Part model, mm, in its own coordinate system. Give positions to 0.01 mm unless a question says otherwise; leave off trailing zeros. Write each loop counter-clockwise with the first axis right and the second up, starting at its lowest first coordinate (ties: lowest second). Pieces come first, ordered by that corner, then holes. Notation, with made-up numbers: M -1,-4.75 L 41,-4.75 A23 cw 41,10.25 Z; hole C -3.75,-6.5 d11. An arc over 180 degrees is marked long. Use a Markdown table: item, result.
```python
from build123d import *

# Parameters (mm, degrees)
F0_R     = 4.222035
F1_DEPTH = 6
F2_DEPTH = 3
F3_SIZE  = 1.5
F4_R     = 1


with BuildPart() as f1:
    # F0 (on Top) → F1 (new body)
    with BuildSketch(Plane.XY):
        with BuildLine():
            Line((31.328976, 34.585057), (-13.897816, 34.585057))
            ThreePointArc((-13.897816, 34.585057), (-27.394685, 43.53433), (-18.671024, 29.890551))
            Line((-18.671024, 29.890551), (-18.671024, -15.414943))
            Line((-18.671024, -15.414943), (31.328976, -15.414943))
            Line((31.328976, -15.414943), (31.328976, 34.585057))
        make_face()
        Polygon((-10.122895, 2.46298), (-0.055609, -7.604307), (-9.207687, -8.519513), (-11.86179, -6.414536), align=None, mode=Mode.SUBTRACT)
        Polygon((11.018406, -7.146703), (-9.685952, 24.921147), (-4.439394, 26.535474), (22.275463, -2.113059), (19.833142, -8.3599), align=None, mode=Mode.SUBTRACT)
        with Locations((-21.591602, 37.633959)):
            Circle(F0_R, mode=Mode.SUBTRACT)
        Polygon((24.128397, 12.799296), (10.983175, 24.906736), (21.130362, 25.598589), (24.704942, 22.254631), align=None, mode=Mode.SUBTRACT)
    extrude(amount=F1_DEPTH)

    # F0 (on Top) → F2 (join)
    with BuildSketch(Plane.XY):
        with BuildLine():
            Line((31.328976, 34.585057), (-13.897816, 34.585057))
            ThreePointArc((-13.897816, 34.585057), (-27.394685, 43.53433), (-18.671024, 29.890551))
            Line((-18.671024, 29.890551), (-18.671024, -15.414943))
            Line((-18.671024, -15.414943), (31.328976, -15.414943))
            Line((31.328976, -15.414943), (31.328976, 34.585057))
        make_face()
        Polygon((-10.122895, 2.46298), (-0.055609, -7.604307), (-9.207687, -8.519513), (-11.86179, -6.414536), align=None, mode=Mode.SUBTRACT)
        Polygon((11.018406, -7.146703), (-9.685952, 24.921147), (-4.439394, 26.535474), (22.275463, -2.113059), (19.833142, -8.3599), align=None, mode=Mode.SUBTRACT)
        with Locations((-21.591602, 37.633959)):
            Circle(F0_R, mode=Mode.SUBTRACT)
        Polygon((24.128397, 12.799296), (10.983175, 24.906736), (21.130362, 25.598589), (24.704942, 22.254631), align=None, mode=Mode.SUBTRACT)
        Polygon((-4.439394, 26.535474), (-9.685952, 24.921147), (11.018406, -7.146703), (19.833142, -8.3599), (22.275463, -2.113059), align=None)
        Polygon((21.130362, 25.598589), (10.983175, 24.906736), (24.128397, 12.799296), (24.704942, 22.254631), align=None)
        Polygon((-9.207687, -8.519513), (-0.055609, -7.604307), (-10.122895, 2.46298), (-11.86179, -6.414536), align=None)
    extrude(amount=F2_DEPTH)

    # F3
    f3_edges = [f1.edges().sort_by_distance(p)[0] for p in [
        (8.918034, 12.211207, 6),
        (-7.062673, 25.72831, 6),
        (0.666227, 8.887222, 6),
        (15.425774, -7.753301, 6),
        (21.054302, -5.23648, 6),
        (22.917652, 23.92661, 6),
        (16.056768, 25.252663, 6),
        (17.555786, 18.853016, 6),
        (24.416669, 17.526963, 6),
        (-5.089252, -2.570663, 6),
        (-10.992342, -1.975778, 6),
        (-10.534738, -7.467025, 6),
        (-4.631648, -8.06191, 6),
    ]]
    chamfer(f3_edges, length=F3_SIZE)

    # F4
    f4_edges = [f1.edges().sort_by_distance(p)[0] for p in [
        (31.328976, 9.585057, 6),
        (6.328976, -15.414943, 6),
        (8.71558, 34.585057, 6),
        (-18.671024, 7.237804, 6),
        (-18.671024, -15.414943, 3),
        (31.328976, -15.414943, 3),
        (31.328976, 34.585057, 3),
    ]]
    fillet(f4_edges, radius=F4_R)


solid = f1.part
```
1. Drill centre lines: L1, parallel to X at y = -4.5, z = 3.75; L2, parallel to Y at x = -3, z = 1; L3, parallel to Z at x = -7.5, y = -5.5. Where is each one in solid material? Low to high.
Findings below:
| item | result |
|---|---|
| L1 | -18.67 to -11.49, -3.16 to 9.31, 21.34 to 31.33 |
| L2 | -15.41 to 34.59 |
| L3 | 0 to 3 |
2. Drop flat-ended pins along their axis: P1, Ø2, axis at y = 12.5, z = 3.5, coming from the -X side; P2, Ø3.5, axis at x = -8.5, y = -4.5, coming from the +Z side; P3, Ø3, axis at x = 6, z = 2.5, coming from the +Y side. Give the stop position or say it passes through.
Findings below:
| item | result |
|---|---|
| P1 | x = -18.67 |
| P2 | z = 3 |
| P3 | y = 34.59 |
3. Cut at B-B, the plane z = 3.75. Give the cut face in (x, y).
Findings below:
| item | result |
|---|---|
| outline | M -18.67,-14.41 A1 ccw -17.67,-15.41 L 30.33,-15.41 A1 ccw 31.33,-14.41 L 31.33,33.59 A1 ccw 30.33,34.59 L -13.9,34.59 A8.28 ccw long -18.67,29.89 Z; hole C -21.59,37.63 d8.44; hole M -11.86,-6.41 L -9.21,-8.52 L -0.06,-7.6 L -10.12,2.46 Z; hole M -9.69,24.92 L 11.02,-7.15 L 19.83,-8.36 L 22.28,-2.11 L -4.44,26.54 Z; hole M 10.98,24.91 L 24.13,12.8 L 24.7,22.25 L 21.13,25.6 Z |
4. Cut at D-D, the plane y = -11. Give the cut face in (x, z), then the cut area to 3 significant figures.
Findings below:
| item | result |
|---|---|
| outline | M -18.67,0 L 31.33,0 L 31.33,5 A1 ccw 30.33,6 L -17.67,6 A1 ccw -18.67,5 Z |
| area | 300 mm2 |
5. Cut at A-A, the plane y = 36. Give the cut face in (x, z).
Findings below:
| item | result |
|---|---|
| outline | M -29.7,0 L -25.48,0 L -25.48,6 L -29.7,6 Z; M -17.7,0 L -13.48,0 L -13.48,6 L -17.7,6 Z |
6. Two-plate mould, pull along X, no slides. Class faces 1 (the flat face through (31.329, 9, 2)), 2 (the flat face through (15.64, -8.53, 5.24)): released by +X, released by -X, zero draft, split by the parting line, or undercut.
Findings below:
| item | result |
|---|---|
| face 1 | released by +X |
| face 2 | undercut |
7. Cut at C-C, the plane x = 18.5. Give the cut face in (y, z).
Findings below:
| item | result |
|---|---|
| outline | M -15.41,0 L 34.59,0 L 34.59,5 A1 ccw 33.59,6 L 26.92,6 L 25.42,4.5 L 25.42,3 L 17.98,3 L 17.98,4.5 L 15.94,6 L 4.14,6 L 1.94,4.5 L 1.94,3 L -8.18,3 L -8.18,4.5 L -9.69,6 L -14.41,6 A1 ccw -15.41,5 Z |
